Could you check a few things on this drawing? It's one solid part, dimensions in mm from its lowest x, y, z. Coordinates: 2 decimals unless noted, no trailing zeros. Loops run counter-clockwise (first coordinate to the right, second up) from the corner with the lowest first, then second, coordinate; pieces in that order, holes last.
1) Imagine slicing it at C-C on y = 62.87. Please give me the cut outline in (x, z).
2) Imagine slicing it at D-D on x = 84.9. Please give me the cut outline in (y, z).
3) If I drill on line 1 along X through (y, z) = (61.5, 0.9) (1 decimal); line 2 along X through (y, z) = (49.5, 0.1); line 3 along Y through (x, z) = (23, 0.5), over which ranges is the centre line in solid material (lowest first)?
4) Imagine slicing it at B-B on z = 0.35. Give the number of separate pieces and of enclosed holes in the cut face, plus the area to 3 significant figures.
5) Imagine slicing it at A-A on x = 54.9. Please give me the cut outline in (y, z).
6) Will these pins go through, and if not, where does the flat tip stop? P1, Ø0.6, axis at x = 106.5, z = 0.5, coming from the +Y side; P2, Ø3.5, axis at x = 84.9, y = 62.87, coming from the -Z side; P3, Ø0.6, axis at y = 52.5, z = 1, coming from the +X side.
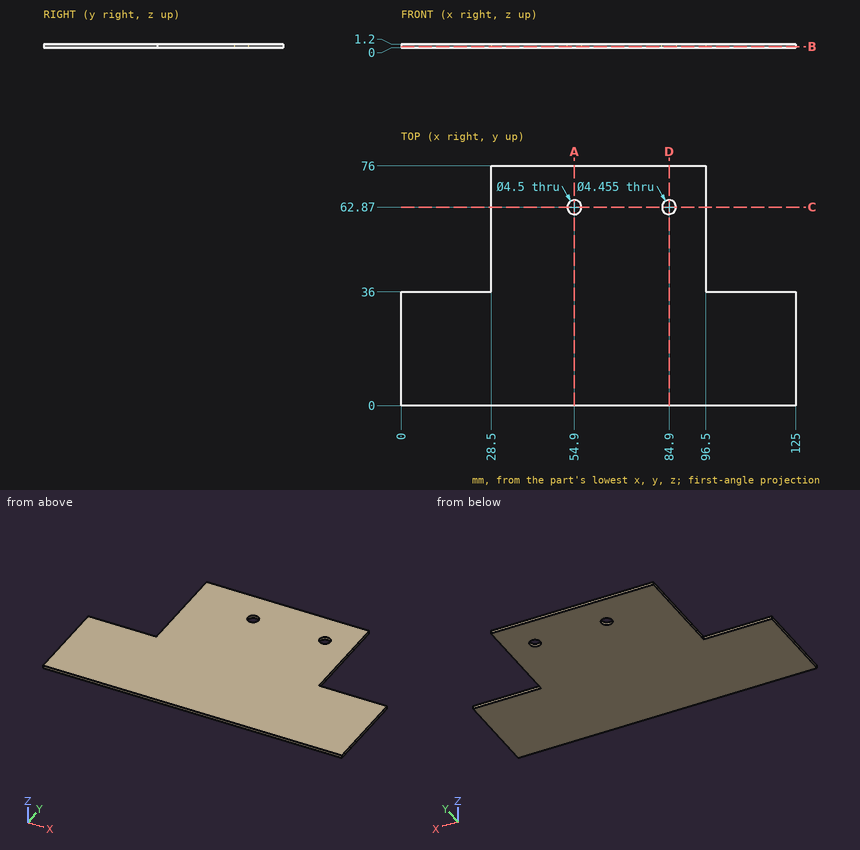
Filled in:
1. outline: (28.5, 0) - (52.65, 0) - (52.65, 1.2) - (28.5, 1.2) - close; (57.15, 0) - (82.67, 0) - (82.67, 1.2) - (57.15, 1.2) - close; (87.13, 0) - (96.5, 0) - (96.5, 1.2) - (87.13, 1.2) - close
2. outline: (0, 0) - (60.64, 0) - (60.64, 1.2) - (0, 1.2) - close; (65.1, 0) - (76, 0) - (76, 1.2) - (65.1, 1.2) - close
3. line 1: x = 28.5 to 53.1, 56.7 to 83.1, 86.7 to 96.5
3. line 2: x = 28.5 to 96.5
3. line 3: y = 0 to 36
4. separate pieces: 1
4. enclosed holes: 2
4. area: 7,190 mm2
5. outline: (0, 0) - (60.62, 0) - (60.62, 1.2) - (0, 1.2) - close; (65.12, 0) - (76, 0) - (76, 1.2) - (65.12, 1.2) - close
6. P1: stops at y = 36
6. P2: passes through
6. P3: stops at x = 96.5
